The figure shows three views and two pictorial views of one solid part (mm, origin at its lowest corner). Answer the questions. A direction names the side the tool comes from. Give positions to 0.01 mm unless a question says otherwise; leave off trailing zeros. Loops run counter-clockwise (first coordinate to the right, second up) from the corner with the lowest first, then second, coordinate; pieces in that order, holes last. Notation, with made-up numbers: (49, 69.25) - (85, 69.25) arc R22 cw to (85, 83.25) - close; hole circle Ø4 at (-30, 14.5). An arc over 180 degrees is marked (long way). Use a Markdown table: item, result. Add a question column.
Item 1: A cutting plane is placed at B-B (y = 22.5). Determine the outline of the cut face in (x, z).
Item 2: For a pull along Y with two mould halves and no side action, classify the marked faces 5, 6, 7 and 8 as +Y half, -Y half, draft (parallel to the pull), parting line (faces both ways), or undercut.
Item 3: Each of these flat-tipped pins is pushed along its axis until it touches: P1, Ø4, axis at x = 44, z = 12, coming from the +Y side; P2, Ø1, axis at y = 23.5, z = 9, coming from the +X side; P3, Ø2.5, axis at x = 11, y = 11, coming from the -Z side; P4, Ø1, axis at y = 1, z = 2, coming from the +X side. Where does it stop, or does it pass through?
Item 4: A cutting plane is placed at C-C (z = 12). Determine the outline of the cut face in (x, y), plus the area to 3 significant figures.
Item 5: Which of the six approach directions +Z, -Z, +X, -X, +Y, -Y give full straight-line access (tool end or side, diameter ignored) to the marked faces 1, 2, 3 and 4?
Item 6: A cutting plane is placed at D-D (y = 6). Determine the outline of the cut face in (x, z), plus the area to 3 significant figures.
Item 7: Consider probe 1 along X at (y, z) = (28.2, 12); probe 2 along Z at (x, y) = (6, 27.45); probe 3 along Y at (x, z) = (12, 5.25). Determine where each line is inside the solid, lowest interval first. Write a range as [from, to].
Item 8: A cutting plane is placed at A-A (x = 44). Determine the outline of the cut face in (y, z).
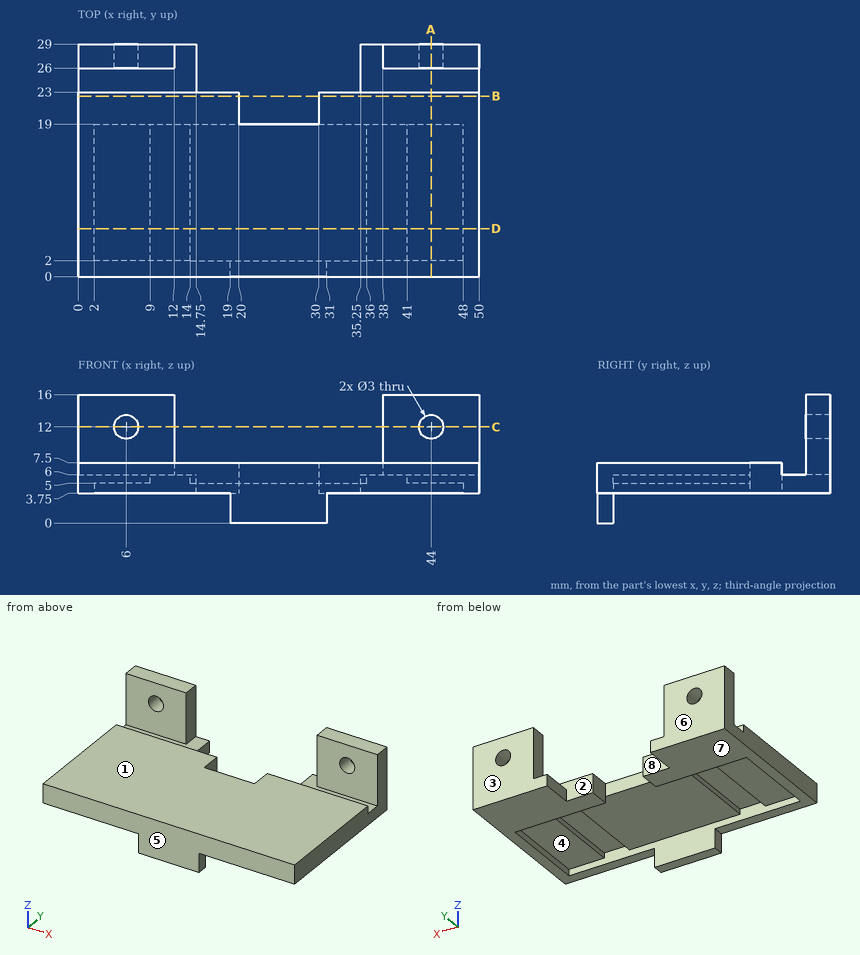
Geometry says:
| question | item | result |
|---|---|---|
| 1 | outline | (0, 3.75) - (20, 3.75) - (20, 7.5) - (0, 7.5) - close; (30, 3.75) - (50, 3.75) - (50, 7.5) - (30, 7.5) - close |
| 2 | face 5 | -Y half |
| 2 | face 6 | +Y half |
| 2 | face 7 | draft |
| 2 | face 8 | undercut |
| 3 | P1 | y = 29 |
| 3 | P2 | through |
| 3 | P3 | z = 6 |
| 3 | P4 | x = 31 |
| 4 | outline | (0, 26) - (4.5, 26) - (4.5, 29) - (0, 29) - close; (7.5, 26) - (12, 26) - (12, 29) - (7.5, 29) - close; (38, 26) - (42.5, 26) - (42.5, 29) - (38, 29) - close; (45.5, 26) - (50, 26) - (50, 29) - (45.5, 29) - close |
| 4 | area | 54.0 mm² |
| 5 | face 1 | +Z, +X, -X, -Y |
| 5 | face 2 | +Z |
| 5 | face 3 | +Z, -Z, +X, -X, +Y |
| 5 | face 4 | -Z |
| 6 | outline | (0, 3.75) - (2, 3.75) - (2, 5) - (9, 5) - (9, 6) - (14, 6) - (14, 5) - (36, 5) - (36, 6) - (41, 6) - (41, 5) - (48, 5) - (48, 3.75) - (50, 3.75) - (50, 7.5) - (0, 7.5) - close |
| 6 | area | 120 mm² |
| 7 | probe 1 | [0, 4.5], [7.5, 12], [38, 42.5], [45.5, 50] |
| 7 | probe 2 | [3.75, 10.5], [13.5, 16] |
| 7 | probe 3 | [0, 2], [19, 29] |
| 8 | outline | (0, 3.75) - (2, 3.75) - (2, 5) - (19, 5) - (19, 3.75) - (29, 3.75) - (29, 10.5) - (26, 10.5) - (26, 6) - (23, 6) - (23, 7.5) - (0, 7.5) - close; (26, 13.5) - (29, 13.5) - (29, 16) - (26, 16) - close |
